Build history of the part. All positions in model axes, mm. Give positions to 0.01 mm unless a question says otherwise; leave off trailing zeros. Order: outer loops, then holes, each group sorted by start corner. A loop starts at its lowest first (then second) coordinate and runs counter-clockwise, first axis right, second up. Notation, with made-up numbers: (83.5, -12) - (110.5, -12) arc R14 ccw to (110.5, 3) - close; hole circle Ø2 at (21.5, 76.5). An arc over 180 degrees is marked (long way). Answer in a Markdown table with one row per item.
Autodesk Inventor part; units mm, degrees
ref_plane "YZ Plane" through (0, 0, 0) normal (1, 0, 0) x (0, 1, 0)
ref_plane "XZ Plane" through (0, 0, 0) normal (0, 1, 0) x (-1, 0, 0)
ref_plane "XY Plane" through (0, 0, 0) normal (0, 0, 1) x (1, 0, 0)
sketch "Szkic3" plane through (0, 0, 0) normal (0, 0, 1) x (1, 0, 0)
  line L0 (-40, -40) -> (40, -40)
  line L1 (40, -40) -> (40, 40)
  line L2 (40, 40) -> (-40, 40)
  line L3 (-40, 40) -> (-40, -40)
  line L4 (-40, -40) -> (40, 40) construction
  line L5 (40, -40) -> (-40, 40) construction
  point P0 (0, 0)
  dimension "d8" = 80
  dimension "d9" = 80
extrude "Wyciągnięcie proste3" add sketch "Szkic3" along normal blind 80
fillet "Zaokrąglenie2" radius 18 2 edges at (0, 40, 0) (0, -40, 0)
fillet "Zaokrąglenie3" radius 40 2 edges at (0, 40, 80) (0, -40, 80)
sketch "Szkic4" plane through (40, -22, 0) normal (1, 0, 0) x (0, 0, -1)
  circle A0 centre (-39.1753, 22) radius 12.5
  point P0 (0, 22)
  dimension "d14" = 25
extrude "Wyciągnięcie proste4" cut sketch "Szkic4" against normal through all
properties part number "jakis_modulxD" material "Stal"
1. Cut at D-D on z = 8.5. Write the cut outline in (x, y).
Check result:
| item | result |
|---|---|
| outline | (-40, -37.29) - (40, -37.29) - (40, 37.29) - (-40, 37.29) - close |
2. Two-plate mould, pull along Z, no slides. Class faces 1 (the face through (0.6, -7.6, 49.1)), 2 (the face through (-1, -40, 29)), 3 (the face through (-1, 0, 0)): +Z half, -Z half, draft (parallel to the pull), parting line (faces both ways), or undercut.
Check result:
| item | result |
|---|---|
| face 1 | undercut |
| face 2 | draft |
| face 3 | -Z half |
3. Cut at B-B on z = 49.5. Write the cut outline in (x, y).
Check result:
| item | result |
|---|---|
| outline | (-40, -38.86) - (40, -38.86) - (40, -7.05) - (-40, -7.05) - close; (-40, 7.05) - (40, 7.05) - (40, 38.86) - (-40, 38.86) - close |
4. Drop flat-ended pins along their axis: P1, Ø2, axis at x = -20.5, y = -18.5, coming from the +Z side; P2, Ø2, axis at x = -23.5, y = -11.5, coming from the +Z side; P3, Ø1, axis at x = -31.5, z = 15, coming from the -Y side. Give the stop position or say it passes through.
Check result:
| item | result |
|---|---|
| P1 | stops at z = 75.97 |
| P2 | stops at z = 78.6 |
| P3 | stops at y = -39.83 |
5. Cut at C-C on y = 5.5. Write the cut outline in (x, z), and give its area (3 significant figures).
Check result:
| item | result |
|---|---|
| outline | (-40, 0) - (40, 0) - (40, 27.95) - (-40, 27.95) - close; (-40, 50.4) - (40, 50.4) - (40, 79.62) - (-40, 79.62) - close |
| area | 4,570 mm² |
6. Probe line 1 (Y direction, x = -16.5, z = 45); line 2 (Y direction, x = -10, z = 17); line 3 (Y direction, x = -27, z = 49). List the from-to ranges inside material, lowest first.
Check result:
| item | result |
|---|---|
| line 1 | y = -39.69 to -11.06, 11.06 to 39.69 |
| line 2 | y = -39.97 to 39.97 |
| line 3 | y = -38.97 to -7.73, 7.73 to 38.97 |
